```python
from build123d import *

# Parameters (mm, degrees)
SKETCH1_R               = 3.81
BOSS_EXTRUDE2_DEPTH     = 228.6
CUT_EXTRUDE1_DEPTH      = 319.859436188
CUT_EXTRUDE1_DEPTH_BACK = 319.859436188
SKETCH3_W               = 209.55
SKETCH3_H               = 457.691503211
SKETCH4_R               = 12.7
BOSS_EXTRUDE3_DEPTH     = 209.55
SCALE1_SCALE            = 2.33


with BuildPart() as part:
    # Sketch1 → Boss-Extrude2 (new body)
    with BuildSketch(Plane(origin=(0, 0, 0), x_dir=(0, 0, -1), z_dir=(1, 0, 0))):
        with BuildLine():
            Line((-203.426935692, 51.985841481), (-25.626935692, 51.985841481))
            Line((-25.626935692, 51.985841481), (43.95726397, 45.89801285))
            Line((43.95726397, 45.89801285), (115.111953895, 32.581774579))
            Line((115.111953895, 32.581774579), (144.05370572, 11.087732787))
            ThreePointArc((144.05370572, 11.087732787), (153.355215288, 6.760397028), (163.609819182, 6.46541568))
            Line((163.609819182, 6.46541568), (178.236347054, 9.045273838))
            ThreePointArc((178.236347054, 9.045273838), (189.948133915, 1.109278265), (182.373529856, -10.839418341))
            Line((182.373529856, -10.839418341), (130.185840083, -23.371799314))
            ThreePointArc((130.185840083, -23.371799314), (120.873250401, -23.847836103), (112.016417856, -20.931081935))
            Line((112.016417856, -20.931081935), (86.281753804, -6.780434321))
            ThreePointArc((86.281753804, -6.780434321), (80.361073143, -4.435827092), (74.043286945, -3.637566412))
            Line((74.043286945, -3.637566412), (-16.495949676, -3.637566412))
            ThreePointArc((-16.495949676, -3.637566412), (-23.382114066, -0.370096092), (-25.206335201, 7.030433588))
            Line((-25.206335201, 7.030433588), (-24.63601234, 9.824433588))
            ThreePointArc((-24.63601234, 9.824433588), (-26.460233475, 17.224963268), (-33.346397865, 20.492433588))
            Line((-33.346397865, 20.492433588), (-174.858415958, 20.492433588))
            Line((-174.858415958, 20.492433588), (-205.966935692, 26.842433588))
            ThreePointArc((-205.966935692, 26.842433588), (-216.062624835, 40.562305299), (-203.426935692, 51.985841481))
        make_face()
        with Locations((-203.426935692, 39.285841481)):
            Circle(SKETCH1_R, mode=Mode.SUBTRACT)
        with Locations((-11.93601234, 5.252433588)):
            Circle(SKETCH1_R, mode=Mode.SUBTRACT)
        with Locations((13.46398766, 22.651433588)):
            Circle(SKETCH1_R, mode=Mode.SUBTRACT)
        with Locations((180.001147709, -0.960278553)):
            Circle(SKETCH1_R, mode=Mode.SUBTRACT)
    extrude(amount=-BOSS_EXTRUDE2_DEPTH)

    # Sketch3 → Cut-Extrude1 (cut, two sides: drawn at the far end of the back side and taken through both)
    with BuildSketch(Plane(origin=(0, 0, 0), x_dir=(1, 0, 0), z_dir=(0, 1, 0)).offset(-CUT_EXTRUDE1_DEPTH_BACK)):
        with Locations((-114.3, -18.881102173)):
            Rectangle(SKETCH3_W, SKETCH3_H)
    extrude(amount=CUT_EXTRUDE1_DEPTH + CUT_EXTRUDE1_DEPTH_BACK, mode=Mode.SUBTRACT)


with BuildPart() as cut_extrude1_piece_1:
    # of the separate pieces the step leaves, piece 1, a body of its own (cut_extrude1_pieces)
    add(part.part.solids().sort_by_distance((0, 51.985841481, 203.426935692))[0])



with BuildPart() as cut_extrude1_piece_2:
    # of the separate pieces the step leaves, piece 2, a body of its own (cut_extrude1_pieces)
    add(part.part.solids().sort_by_distance((-219.075, 51.985841481, 203.426935692))[0])


with BuildPart() as cut_extrude1_piece_1_1:
    add(cut_extrude1_piece_1.part)

    add(cut_extrude1_piece_2.part)  # Boss-Extrude3 merges Cut-Extrude1 piece 2
    # Sketch4 → Boss-Extrude3 (add)
    with BuildSketch(Plane(origin=(-219.075, 0, 0), x_dir=(0, 0, -1), z_dir=(1, 0, 0))):
        with Locations(Location((102.411953895, 18.161886375, 0), (0, 0, 180))):
            Circle(SKETCH4_R)
    extrude(amount=BOSS_EXTRUDE3_DEPTH)


with BuildPart() as cut_extrude1_piece_1_2:
    # Scale1: scaled about (-114.3, 21.499691493, -25.72204861)
    add(cut_extrude1_piece_1_1.part.scale(SCALE1_SCALE).moved(Location((152.019, -28.594589686, 34.210324651))))


solid = cut_extrude1_piece_1_2.part
```
For this review, take the finished solid that the model builds, in its own axes (mm). A direction names the side the tool comes from. Coordinates: 2 decimals unless noted, no trailing zeros. Order: outer loops, then holes, each group sorted by start corner. A loop starts at its lowest first (then second) coordinate and runs counter-clockwise, first axis right, second up. Notation, with made-up numbers: (-21.75, 52) -> (31.25, 52) arc R22 cw to (31.25, 67) -> close; hole circle Ø2 at (53, 84.25). An arc over 180 degrees is marked (long way). Answer as CSV lines item,"result".
Q1. We need section B-B (y = -63). State the section outline as (x, z) points.
Model answer:
outline,"(-380.62, -352.62) -> (-358.43, -352.62) -> (-358.43, -200.67) -> (-380.62, -200.67) -> close; (129.83, -352.62) -> (152.02, -352.62) -> (152.02, -200.67) -> (129.83, -200.67) -> close"
Q2. Wall thickness on line 1 along X through (y, z) = (-53.5, -314.5); line 2 along Z through (x, y) = (-173, 41); line 3 along Z through (x, y) = (-293, 31): over which ranges is each line inside the solid? List them lowest first. Write a range as [from, to].
Model answer:
line 1,"x = [-380.62, -358.43], [129.83, 152.02]"
line 2,"z = [-215.88, -192.94]"
line 3,"z = [-228.43, -180.39]"
Q3. We need section A-A (z = 189). State the section outline as (x, y) points, plus the area to 3 significant figures.
Model answer:
outline,"(-380.62, 19.15) -> (-358.43, 19.15) -> (-358.43, 92.53) -> (-380.62, 92.53) -> close; (129.83, 19.15) -> (152.02, 19.15) -> (152.02, 92.53) -> (129.83, 92.53) -> close"
area,"3,260 mm2"
Q4. We need section C-C (z = -206.5). State the section outline as (x, y) points.
Model answer:
outline,"(-380.62, -66.21) -> (-358.43, -66.21) -> (-358.43, -15.79) -> (129.83, -15.79) -> (129.83, -66.21) -> (152.02, -66.21) -> (152.02, 52.47) -> (129.83, 52.47) -> (129.83, 43.24) -> (-358.43, 43.24) -> (-358.43, 52.47) -> (-380.62, 52.47) -> close"
Q5. For faces 4 (the face through (-380.619, 25, 58)), 5 (the face through (141, -37.07, -34)), list the 3-axis set-ups (+Z, -Z, +X, -X, +Y, -Y) from which the entire face can be reached by the end or side of a thin tool; tool diameter is ignored.
Model answer:
face 4,"+Z, -Z, -X, +Y, -Y"
face 5,"+Z, +X, -X, -Y"
Q6. We need section D-D (x = 87). State the section outline as (y, z) points, plus the area to 3 significant figures.
Model answer:
outline,"circle Ø59.18 at (13.72, -204.41)"
area,"2,750 mm2"
Q7. Draft analysis for pull direction Y (two halves, no side actions). For faces 1 (the face through (141.08, 65.61, 499.73)), 2 (the face through (-369.367, 26.447, 477.364)), 3 (the face through (-369.37, -25.51, -408.26)), state which applies: released by +Y, released by -Y, zero draft, split by the parting line, or undercut.
Model answer:
face 1,"undercut"
face 2,"released by -Y"
face 3,"split by the parting line"
Q8. Clearance check with flat-ended pins moving along their axes: pin 1 Ø6.5 at (x, z) = (145.5, -39) entering from -Y; pin 2 Ø14 at (y, z) = (-30.83, -385.19) entering from +X; pin 3 Ø10 at (x, z) = (-156, -228.5) entering from +Y; pin 4 Ø10 at (x, y) = (31.5, 37) entering from -Z. State where each tip first meets the part, or that it passes through.
Model answer:
pin 1,"stops at y = -37.07"
pin 2,"passes through"
pin 3,"stops at y = 36.33"
pin 4,"stops at z = -227.68"
